from build123d import *

# Parameters (mm, degrees)
F0_R     = 14.532496
F1_DEPTH = 135.128
F2_W     = 21.599732
F2_H     = 69.967128
F3_DEPTH = 24.638
F5_DEPTH = 52.07
F6_R     = 12.97612
F7_DEPTH = 132.334


with BuildPart() as f1:
    # F0 (on Front) → F1 (new body)
    with BuildSketch(Plane.XZ):
        Circle(F0_R)
    extrude(amount=F1_DEPTH)

    # F2 (on Top) → F3 (join)
    with BuildSketch(Plane.XY):
        Rectangle(F2_W, F2_H)
    extrude(amount=F3_DEPTH)

    # F4 (on Top) → F5 (join)
    with BuildSketch(Plane.XY):
        Polygon((-19.11266, 0), (0, 0), (0, 24.325365), (-19.11266, 24.325365), (-19.11266, 3.464378), align=None)
    extrude(amount=-F5_DEPTH)

    # F6 (on Front) → F7 (join)
    with BuildSketch(Plane.XZ):
        with Locations((-24.016608, 0)):
            Circle(F6_R)
    extrude(amount=F7_DEPTH)


solid = f1.part
The model under review builds one solid part; all positions refer to its coordinate system, in mm. A direction names the side the tool comes from. Round coordinates to 2 decimals unless told otherwise and drop trailing zeros. Write each loop counter-clockwise with the first axis right and the second up, starting at its lowest first coordinate (ties: lowest second). Pieces come first, ordered by that corner, then holes. Notation, with made-up numbers: (3, 15.25) - (48, 15.25) arc R26 ccw to (48, 41.25) - close; hole circle Ø2 at (40.5, 56.5). An arc over 180 degrees is marked (long way). One line per item, written item: value. Start each with the question number.
1. Clearance check with flat-ended pins moving along their axes: P1, Ø9.5, axis at x = -11.5, z = -27.5, coming from the +Y side; P2, Ø19.5, axis at y = 8.5, z = -35.5, coming from the +X side; P3, Ø2, axis at x = 7.5, z = -11.5, coming from the +Y side. State where each tip first meets the part, or that it passes through.
2. Consider section B-B on z = -9. Write out the cut boundary in (x, y), and give its area (3 significant figures).
3. To check wall thickness, follow L1, parallel to Y at x = -19.5, z = 6.5; L2, parallel to X at y = -19.5, z = -9; L3, parallel to Z at x = -6.5, y = -2. State the ranges of each line that lie inside material, in increasing order. Write a range as from..to.
4. Consider section C-C on x = -3.5. Write out the cut boundary in (y, z).
5. The part is to be moulded in two halves that separate along X. For faces 4 (the face through (-36.984, -65.241, 0.472)), 5 (the face through (-19.113, 12, -26)), 6 (the face through (0, -135.128, 0)), say which applies: released by +X, released by -X, zero draft, split by the parting line, or undercut.
6. Consider section A-A on y = -10.5. Write out the cut boundary in (x, z) (1 decimal).
7. Machinability: for faces 1 (the face through (0, 12, -26)), 2 (the face through (-9, 24.325, -26)), 3 (the face through (-15, 12, 0)), which of the approach directions +Z, -Z, +X, -X, +Y, -Y give a long, thin tool a straight path to every point of the face, cutting with its end or side? Answer none if there is none.
8. Consider section D-D on z = -38.5. Write out the cut boundary in (x, y).
Checks:
1. P1: stops at y = 24.33
1. P2: stops at x = 0
1. P3: stops at y = 0
2. outline: (-33.36, -132.33) - (-14.67, -132.33) - (-14.67, 0) - (-11.41, 0) - (-11.41, -135.13) - (11.41, -135.13) - (11.41, 0) - (0, 0) - (0, 24.33) - (-19.11, 24.33) - (-19.11, 0) - (-33.36, 0) - close
2. area: 6,020 mm^2
3. L1: y = -132.33..0
3. L2: x = -33.36..-14.67, -11.41..11.41
3. L3: z = -13..24.64
4. outline: (-135.13, -14.1) - (0, -14.1) - (0, -52.07) - (24.33, -52.07) - (24.33, 0) - (34.98, 0) - (34.98, 24.64) - (-34.98, 24.64) - (-34.98, 14.1) - (-135.13, 14.1) - close
5. face 4: undercut
5. face 5: released by -X
5. face 6: zero draft
6. outline: (-12.9, -6.7) arc R14.5 ccw (long way) to (10.8, 9.7) - (10.8, 24.6) - (-10.8, 24.6) - (-10.8, 9.7) arc R14.5 ccw to (-12.9, 6.7) arc R13 ccw (long way) to start
7. face 1: -Z, +X, +Y
7. face 2: -Z, +X, -X, +Y
7. face 3: +Z, -X, +Y
8. outline: (-19.11, 0) - (0, 0) - (0, 24.33) - (-19.11, 24.33) - close
